Read the model definition and answer for the solid it produces. Units are mm, in the model's axes. A direction names the side the tool comes from. Round coordinates to 2 decimals unless told otherwise and drop trailing zeros. Order: outer loops, then holes, each group sorted by start corner. A loop starts at its lowest first (then second) coordinate and runs counter-clockwise, first axis right, second up.
from build123d import *

# Parameters (mm, degrees)
POCKET002_DEPTH = 10
SKETCH006_R     = 4
POCKET003_DEPTH = 5


with BuildPart() as part:
    # Sketch004 → Revolution (revolve)
    with BuildSketch(Plane.XY):
        with BuildLine():
            ThreePointArc((15.999978, -20), (18.343131, -25.656862), (24, -28))
            Line((24, -30), (24, -28))
            ThreePointArc((13.999978, -20), (16.928918, -27.071076), (24, -30))
            Line((13.999978, -20), (13.999978, -18))
            ThreePointArc((13.999978, -18), (13.414191, -16.585786), (11.999978, -16))
            Line((11.999978, -16), (0, -16))
            Line((0, -16), (0, -14))
            Line((0, -14), (11.999978, -14))
            ThreePointArc((15.999978, -18), (14.828405, -15.171573), (11.999978, -14))
            Line((15.999978, -18), (15.999978, -20))
        make_face()
    revolve(axis=Axis((0, 0, 0), (0, 1, 0)))

    # Sketch005 (on DatumPlane) → Pocket002 (cut)
    with BuildSketch(Plane(origin=(0, -30, 0), x_dir=(0, 0, 1), z_dir=(0, -1, 0))):
        with BuildLine():
            ThreePointArc((12.353429, -20.576511), (22.552623, -8.208483), (22.689602, 7.82189))
            Line((22.689602, 7.82189), (3.322315, -1.209224))
            Line((3.322315, -1.209224), (12.353429, -20.576511))
        make_face()
        with BuildLine():
            ThreePointArc((20.576511, 12.353429), (8.208483, 22.552623), (-7.82189, 22.689602))
            Line((-7.82189, 22.689602), (1.209224, 3.322315))
            Line((20.576511, 12.353429), (1.209224, 3.322315))
        make_face()
        with BuildLine():
            ThreePointArc((-12.353429, 20.576511), (-22.552623, 8.208483), (-22.689602, -7.82189))
            Line((-22.689602, -7.82189), (-3.322315, 1.209224))
            Line((-3.322315, 1.209224), (-12.353429, 20.576511))
        make_face()
        with BuildLine():
            ThreePointArc((-20.576511, -12.353429), (-8.208483, -22.552623), (7.82189, -22.689602))
            Line((7.82189, -22.689602), (-1.209224, -3.322315))
            Line((-1.209224, -3.322315), (-20.576511, -12.353429))
        make_face()
    extrude(amount=-POCKET002_DEPTH, mode=Mode.SUBTRACT)

    # Sketch006 (on Face30 of Pocket002) → Pocket003 (cut)
    with BuildSketch(Plane.XZ.offset(16)):
        Circle(SKETCH006_R)
    extrude(amount=POCKET003_DEPTH, mode=Mode.SUBTRACT)


solid = part.part
Q1. A cutting plane is placed at C-C, the plane x = 0. Give the vertices of the cut face in (y, z).
Outcome:
outline: (-20, -16) - (-18, -16) arc R4 ccw to (-14, -12) - (-14, 12) arc R4 ccw to (-18, 16) - (-20, 16) - (-20, 14) - (-18, 14) arc R2 cw to (-16, 12) - (-16, -12) arc R2 cw to (-18, -14) - (-20, -14) - close
Q2. Straight lines are drawn through the part: probe 1 along X at (y, z) = (-19.25, 0); probe 2 along Y at (x, z) = (7, 9.5). For each, find the intervals that lie inside material, in ascending order.
Outcome:
probe 1: x = -16 to -14, 14 to 16
probe 2: y = -16 to -14
Q3. Flat-ended cylindrical pins translate along their axes: pin 1 (5 mm diameter, centred on y = -18, z = -5.5, fed in from +X); pin 2 (2.5 mm diameter, centred on x = -0.5, z = -12, fed in from -Y); pin 3 (1 mm diameter, centred on x = 2.5, z = 17.5, fed in from +Y); pin 4 (3 mm diameter, centred on x = -15.5, y = -18, fed in from -Z). Find the tip coordinate at first contact, or state that the pin passes through.
Outcome:
pin 1: stops at x = 15.72
pin 2: stops at y = -16.45
pin 3: passes through
pin 4: stops at z = -7.75
Q4. A cutting plane is placed at D-D, the plane y = -21.5. Give the vertices of the cut face in (x, z), plus the area to 3 significant figures.
Outcome:
outline: (-15.51, -4.47) arc R16.14 ccw to (-13.4, -9.01) - (-11.53, -8.14) arc R14.11 cw to (-13.65, -3.6) - close; (-9.01, 13.4) - (-8.14, 11.53) arc R14.11 cw to (-3.6, 13.65) - (-4.47, 15.51) arc R16.14 ccw to start; (3.6, -13.65) - (4.47, -15.51) arc R16.14 ccw to (9.01, -13.4) - (8.14, -11.53) arc R14.11 cw to start; (11.53, 8.14) arc R14.11 cw to (13.65, 3.6) - (15.51, 4.47) arc R16.14 ccw to (13.4, 9.01) - close
area: 40.8 mm2
Q5. For faces 1 (the face through (-17.12, -26.134, -5.225)), 2 (the face through (5.225, -26.134, -17.12)), 3 (the face through (-14.964, -25.764, -9.736)), 4 (the face through (-3.03, -18.99, 13.67)), determine the directions among +Z, -Z, +X, -X, +Y, -Y from which every point of the face is accessible in a straight line to the end or side of a thin tool.
Outcome:
face 1: +Z, -X, -Y
face 2: -Z, -X, -Y
face 3: -Z, +X, -Y
face 4: -Y
Q6. A cutting plane is placed at B-B, the plane z = 0. Give the vertices of the cut face in (x, y).
Outcome:
outline: (-16, -20) - (-14, -20) - (-14, -18) arc R2 cw to (-12, -16) - (12, -16) arc R2 cw to (14, -18) - (14, -20) - (16, -20) - (16, -18) arc R4 ccw to (12, -14) - (-12, -14) arc R4 ccw to (-16, -18) - close
Q7. A cutting plane is placed at A-A, the plane y = -26.5. Give the vertices of the cut face in (x, z).
Outcome:
outline: (-18.43, -5.84) arc R19.34 ccw to (-16.32, -10.37) - (-13.63, -9.12) arc R16.4 cw to (-15.75, -4.58) - close; (-10.37, 16.32) - (-9.12, 13.63) arc R16.4 cw to (-4.58, 15.75) - (-5.84, 18.43) arc R19.34 ccw to start; (4.58, -15.75) - (5.84, -18.43) arc R19.34 ccw to (10.37, -16.32) - (9.12, -13.63) arc R16.4 cw to start; (13.63, 9.12) arc R16.4 cw to (15.75, 4.58) - (18.43, 5.84) arc R19.34 ccw to (16.32, 10.37) - close
